from build123d import *

# Parameters (mm, degrees)
SKETCH1_R           = 2.5
BOSS_EXTRUDE1_DEPTH = 60
FILLET1_R           = 1.47
SKETCH2_R           = 1.5
CUT_EXTRUDE1_DEPTH  = 63.395592793


with BuildPart() as part:
    # Sketch1 → Boss-Extrude1 (new body)
    with BuildSketch(Plane.XY):
        Polygon((2.860553032, 3.9), (6, 7.039446968), (6, 8.2), (3.1, 8.2), (3.1, 10), (10, 10), (10, 3.1), (8.2, 3.1), (8.2, 6), (7.039446968, 6), (3.9, 2.860553032), (3.9, 0), (3.9, -2.860553032), (7.039446968, -6), (8.2, -6), (8.2, -3.1), (10, -3.1), (10, -10), (3.1, -10), (3.1, -8.2), (6, -8.2), (6, -7.039446968), (2.860553032, -3.9), (0, -3.9), (-2.860553032, -3.9), (-6, -7.039446968), (-6, -8.2), (-3.1, -8.2), (-3.1, -10), (-10, -10), (-10, -3.1), (-8.2, -3.1), (-8.2, -6), (-7.039446968, -6), (-3.9, -2.860553032), (-3.9, 0), (-3.9, 2.860553032), (-7.039446968, 6), (-8.2, 6), (-8.2, 3.1), (-10, 3.1), (-10, 10), (-3.1, 10), (-3.1, 8.2), (-6, 8.2), (-6, 7.039446968), (-2.860553032, 3.9), (0, 3.9), align=None)
        Circle(SKETCH1_R, mode=Mode.SUBTRACT)
    extrude(amount=BOSS_EXTRUDE1_DEPTH)

    # Fillet1
    fillet1_edges = [part.edges().sort_by_distance(p)[0] for p in [
        (10, -10, 30),
        (-10, -10, 30),
        (-10, 10, 30),
        (10, 10, 30),
    ]]
    fillet(fillet1_edges, radius=FILLET1_R)

    # Sketch2 → Cut-Extrude1 (cut, through all)
    with BuildSketch(Plane(origin=(3.9, 0, 0), x_dir=(0, 0, -1), z_dir=(1, 0, 0))):
        with Locations(Location((-50, 0, 0), (0, 0, 90))):
            Circle(SKETCH2_R)
        with Locations(Location((-40, 0, 0), (0, 0, 90))):
            Circle(SKETCH2_R)
        with Locations(Location((-30, 0, 0), (0, 0, 90))):
            Circle(SKETCH2_R)
        with Locations(Location((-20, 0, 0), (0, 0, 90))):
            Circle(SKETCH2_R)
    extrude(amount=-CUT_EXTRUDE1_DEPTH, mode=Mode.SUBTRACT)


solid = part.part
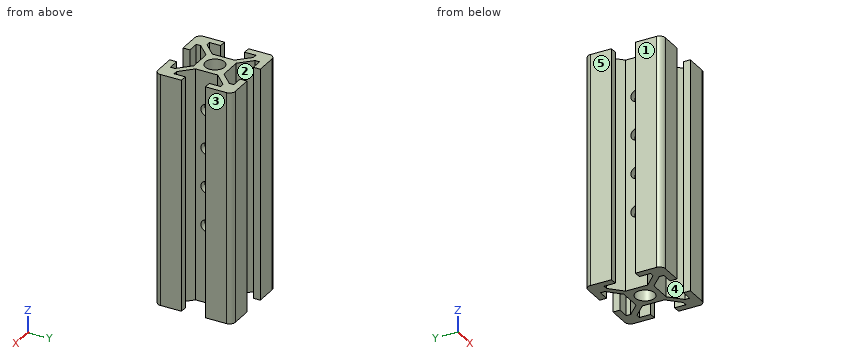
Work out the finished part from the listing and answer in its coordinate system (mm). Face numbers are marked on the shaded views. A direction names the side the tool comes from. Give positions to 0.01 mm unless a question says otherwise; leave off trailing zeros. Loops run counter-clockwise (first coordinate to the right, second up) from the corner with the lowest first, then second, coordinate; pieces in that order, holes last. Notation, with made-up numbers: (32.5, -38) -> (72.5, -38) arc R17 ccw to (72.5, -24) -> close; hole circle Ø8 at (84.25, 72). An arc over 180 degrees is marked (long way). Use a Markdown table: item, result. Add a question column.
1) The part is cut by section B-B, the plane y = 0. Count the separate pieces of the cut face and the enclosed holes in it, plus the area to 3 significant figures.
2) Each of these flat-tipped pins is pushed along its axis until it touches: P1, Ø1, axis at x = -1.5, z = 30, coming from the +Y side; P2, Ø3.5, axis at y = 0, z = 20, coming from the -X side; P3, Ø1.7, axis at x = 1.5, z = 30.5, coming from the -Y side. Where does it stop, or does it pass through?
3) Consider line 1 along Z through (x, y) = (-2.75, 0); line 2 along Y through (x, z) = (2.5, 30); line 3 along Y through (x, z) = (-3.3, 50). Determine where each line is inside the solid, lowest interval first.
4) For a pull along X with two mould halves and no side action, classify the marked faces 3, 4 and 5 as +X half, -X half, draft (parallel to the pull), parting line (faces both ways), or undercut.
5) Which of the six approach directions +Z, -Z, +X, -X, +Y, -Y give full straight-line access (tool end or side, diameter ignored) to the marked faces 1 and 2?
6) The part is cut by section A-A, the plane x = 0. Determine the outline of the cut face in (y, z), plus the area to 3 significant figures.
Reported:
| question | item | result |
|---|---|---|
| 1 | separate pieces | 10 |
| 1 | enclosed holes | 0 |
| 1 | area | 134 mm^2 |
| 2 | P1 | stops at y = 3.9 |
| 2 | P2 | stops at x = -3.9 |
| 2 | P3 | stops at y = -3.9 |
| 3 | line 1 | z = 0 to 18.5, 21.5 to 28.5, 31.5 to 38.5, 41.5 to 48.5, 51.5 to 60 |
| 3 | line 2 | y = -3.9 to -1.5, 1.5 to 3.9 |
| 3 | line 3 | y = -10 to -8.2, -4.34 to -1.5, 1.5 to 4.34, 8.2 to 10 |
| 4 | face 3 | +X half |
| 4 | face 4 | undercut |
| 4 | face 5 | -X half |
| 5 | face 1 | +Z, -Z, -X, +Y, -Y |
| 5 | face 2 | +Z, -Z |
| 6 | outline | (-3.9, 0) -> (-2.5, 0) -> (-2.5, 60) -> (-3.9, 60) -> close; (2.5, 0) -> (3.9, 0) -> (3.9, 60) -> (2.5, 60) -> close |
| 6 | area | 168 mm^2 |
